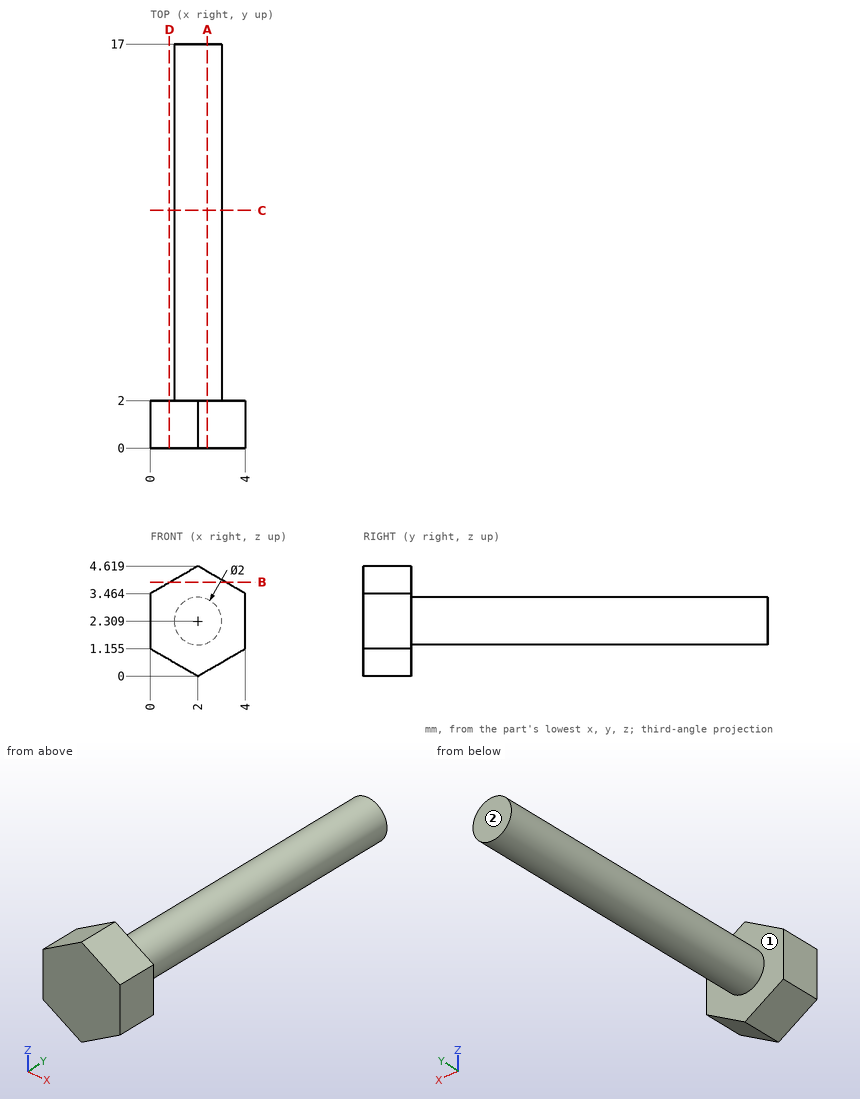
Print and shaded views of the part. All mm, measured from the part's lowest x, y and z. A direction names the side the tool comes from. Coordinates: 2 decimals unless noted, no trailing zeros. Loops run counter-clockwise (first coordinate to the right, second up) from the corner with the lowest first, then second, coordinate; pieces in that order, holes last. Notation, with made-up numbers: (66, 59.5) -> (74, 59.5) arc R24 cw to (74, 94.5) -> close; hole circle Ø9 at (22.25, -33.75). An arc over 180 degrees is marked (long way). Use one line per item in the form item = value. Start each with the question number.
(1) Cut at B-B on z = 3.95. Give the cut face in (x, y).
(2) Tool access for the marked faces 1 and 2: list every direction of +Z, -Z, +X, -X, +Y, -Y with a clear straight run to the whole face (end or side of a thin tool).
(3) Cut at D-D on x = 0.8. Give the cut face in (y, z).
(4) Cut at C-C on y = 10. Give the cut face in (x, z).
(5) Flat gauge pins, fed straight in: pin 1 (1.5 mm diameter, centred on y = 3.5, z = 1, fed in from -X); pin 2 (1.5 mm diameter, centred on x = 3.5, y = 9, fed in from -Z). Where does each tip first touch, or does it go through?
(6) Cut at A-A on x = 2.4. Give the cut face in (y, z), and give its area (3 significant figures).
(7) Probe probe 1 along Y at (x, z) = (2.15, 3.7); probe 2 along X at (y, z) = (6.5, 1.65); probe 3 along X at (y, z) = (15.5, 2.1). List the from-to ranges inside material, lowest first. Write a range as from..to.
Values:
q1.outline = (0.84, 0) -> (3.16, 0) -> (3.16, 2) -> (0.84, 2) -> close
q2.face_1 = +Y
q2.face_2 = +Z, -Z, +X, -X, +Y
q3.outline = (0, 0.69) -> (2, 0.69) -> (2, 3.93) -> (0, 3.93) -> close
q4.outline = circle Ø2 at (2, 2.31)
q5.pin_1 = 1.17
q5.pin_2 = 1.65
q6.outline = (0, 0.23) -> (2, 0.23) -> (2, 1.39) -> (17, 1.39) -> (17, 3.23) -> (2, 3.23) -> (2, 4.39) -> (0, 4.39) -> close
q6.area = 35.8 mm2
q7.probe_1 = 0..2
q7.probe_2 = 1.25..2.75
q7.probe_3 = 1.02..2.98
